Can you work these out from the model? Positions are in its coordinate system, mm. Face numbers are marked on the shaded views. Round coordinates to 2 decimals unless told otherwise and drop trailing zeros. Loops run counter-clockwise (first coordinate to the right, second up) from the corner with the lowest first, then second, coordinate; pieces in that order, holes last.
(1) Will these pins go through, and if not, where does the flat tip stop? pin 1 Ø3 at (x, z) = (2.5, -41) entering from +Y; pin 2 Ø1 at (x, z) = (-5, -10.5) entering from -Y; pin 3 Ø2 at (y, z) = (2, -13.5) entering from -X.
(2) Thinking about a two-plate mould opening in Y: for the marked faces 1, 2 and 3, which applies, released by +Y, released by -Y, zero draft, split by the parting line, or undercut?
(3) I want a section at A-A on z = -6. Write out the boundary of the cut face in (x, y).
(4) I want a section at D-D on z = -43. Write out the boundary of the cut face in (x, y).
(5) If I drill on line 1 along Y through (x, z) = (0, -13); line 2 along Z through (x, y) = (1.5, 6.25), over which ranges is the centre line in solid material (lowest first)?
(6) I want a section at B-B on x = 0. Write out the boundary of the cut face in (y, z), plus the area to 3 significant figures.
Autodesk Inventor part; units mm, degrees
ref_plane "YZ Plane" through (0, 0, 0) normal (1, 0, 0) x (0, 1, 0)
ref_plane "XZ Plane" through (0, 0, 0) normal (0, 1, 0) x (-1, 0, 0)
ref_plane "XY Plane" through (0, 0, 0) normal (0, 0, 1) x (1, 0, 0)
sketch "Skizze2" plane through (0, 0, 0) normal (0, 1, 0) x (-1, 0, 0)
  line L0 (0, 0) -> (6.5, 0)
  line L1 (6.5, 0) -> (6.5, -34)
  line L2 (6.5, -34) -> (4, -34)
  line L3 (4, -34) -> (4, -74)
  line L4 (4, -74) -> (0, -74)
  line L5 (0, -74) -> (0, 0)
  dimension "d3" = 13
  dimension "d4" = 8
  dimension "d5" = 34
  dimension "d6" = 40
revolve "Umdrehung1" add sketch "Skizze2" angle 360 about axis through (0, 0, -74) along (0, 0, 1)
chamfer "Fasen1" distance 0.6 angle 45 1 edges at (4, 0, -74)
sketch "Skizze3" plane through (0, 0, 0) normal (0, 0, 1) x (1, 0, 0)
  circle A0 centre (0, 0) radius 6.5
  point P0 (0, 0)
hole "Bohrung1" at (0, 0, 0) direction (0, 0, -1) diameter 6 depth 34
properties part number "202 Welle" material "Aluminium 6061"
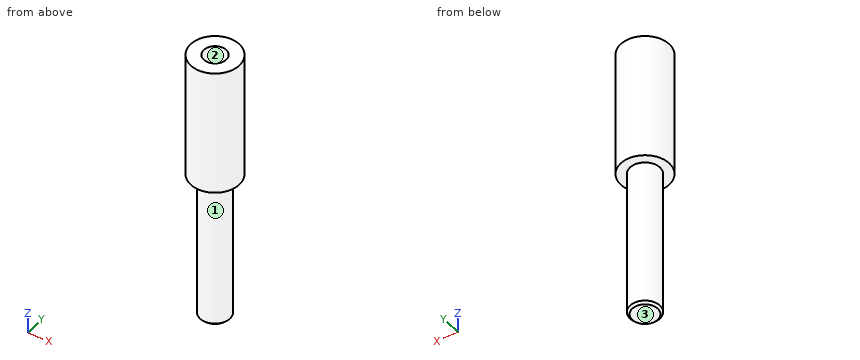
Filled sheet:
1. pin 1: stops at y = 3.87
1. pin 2: stops at y = -4.69
1. pin 3: stops at x = -6.42
2. face 1: split by the parting line
2. face 2: undercut
2. face 3: zero draft
3. outline: circle Ø13 at (0, 0); hole circle Ø6 at (0, 0)
4. outline: circle Ø8 at (0, 0)
5. line 1: y = -6.5 to -3, 3 to 6.5
5. line 2: z = -34 to 0
6. outline: (-6.5, -34) - (-4, -34) - (-4, -73.4) - (-3.4, -74) - (3.4, -74) - (4, -73.4) - (4, -34) - (6.5, -34) - (6.5, 0) - (3, 0) - (3, -34) - (-3, -34) - (-3, 0) - (-6.5, 0) - close
6. area: 558 mm2
